```python
from build123d import *

# Parameters (mm, degrees)
SKETCH1_W           = 35
SKETCH1_H           = 48
BOSS_EXTRUDE1_DEPTH = 4
SKETCH2_W           = 35
SKETCH2_H           = 48
SKETCH2_W_2         = 31
SKETCH2_H_2         = 44
BOSS_EXTRUDE2_DEPTH = 5.5
SKETCH3_W           = 10
SKETCH3_H           = 6
SKETCH3_W_2         = 5.25
SKETCH3_H_2         = 8
BOSS_EXTRUDE3_DEPTH = 5.5
SKETCH4_W           = 20.5
SKETCH4_H           = 5.5
CUT_EXTRUDE1_DEPTH  = 3
CUT_EXTRUDE2_DEPTH  = 2
CUT_EXTRUDE3_REACH  = 33.185
SKETCH7_W           = 5.25
SKETCH7_H           = 3.1
CUT_EXTRUDE4_START  = 9.5
SKETCH8_R           = 1.55
CUT_EXTRUDE4_DEPTH  = 5.5
SKETCH5_W           = 5
SKETCH5_H           = 5
CUT_EXTRUDE5_DEPTH  = 2


with BuildPart() as part:
    # Sketch1 → Boss-Extrude1 (new body)
    with BuildSketch(Plane(origin=(0, 0, 0), x_dir=(1, 0, 0), z_dir=(0, 1, 0))):
        Rectangle(SKETCH1_W, SKETCH1_H)
    extrude(amount=BOSS_EXTRUDE1_DEPTH)

    # Sketch2 → Boss-Extrude2 (add)
    with BuildSketch(Plane(origin=(0, 4, 0), x_dir=(1, 0, 0), z_dir=(0, 1, 0))):
        Rectangle(SKETCH2_W, SKETCH2_H)
        with Locations((0, 1)):
            Rectangle(SKETCH2_W_2, SKETCH2_H_2, mode=Mode.SUBTRACT)
    extrude(amount=BOSS_EXTRUDE2_DEPTH)

    # Sketch3 → Boss-Extrude3 (add)
    with BuildSketch(Plane(origin=(0, 4, 0), x_dir=(1, 0, 0), z_dir=(0, 1, 0))):
        with Locations((0, 20)):
            Rectangle(SKETCH3_W, SKETCH3_H)
        with Locations((-12.875, -17)):
            Rectangle(SKETCH3_W_2, SKETCH3_H_2)
        with Locations((12.875, -17)):
            Rectangle(SKETCH3_W_2, SKETCH3_H_2)
    extrude(amount=BOSS_EXTRUDE3_DEPTH)

    # Sketch4 → Cut-Extrude1 (cut)
    with BuildSketch(Plane.XY.offset(24)):
        with Locations((0, 6.75)):
            Rectangle(SKETCH4_W, SKETCH4_H)
    extrude(amount=-CUT_EXTRUDE1_DEPTH, mode=Mode.SUBTRACT)

    # Sketch6 → Cut-Extrude2 (cut)
    with BuildSketch(Plane(origin=(0, 0, -24), x_dir=(-1, 0, 0), z_dir=(0, 0, -1))):
        with BuildLine():
            ThreePointArc((-12.93428015, 9.5), (-10, 5.4), (-7.06571985, 9.5))
            Line((-7.06571985, 9.5), (-12.93428015, 9.5))
        make_face()
        with BuildLine():
            Line((12.93428015, 9.5), (7.06571985, 9.5))
            ThreePointArc((7.06571985, 9.5), (10, 5.4), (12.93428015, 9.5))
        make_face()
    extrude(amount=-CUT_EXTRUDE2_DEPTH, mode=Mode.SUBTRACT)

    # Cut-Extrude3: up to this face of the body (flat: up to its plane)
    cut_extrude3_end = Plane(part.part.faces().sort_by_distance((0, 0, 0))[0])
    # Sketch7 → Cut-Extrude3 (cut, up to the picked face)
    with BuildSketch(Plane(origin=(0, 9.5, 0), x_dir=(1, 0, 0), z_dir=(0, 1, 0)), mode=Mode.PRIVATE) as cut_extrude3_sk1:
        with Locations((-12.875, -13.55)):
            Rectangle(SKETCH7_W, SKETCH7_H)
    cut_extrude3_tool1 = split(extrude(cut_extrude3_sk1.sketch, amount=-CUT_EXTRUDE3_REACH, mode=Mode.PRIVATE), bisect_by=cut_extrude3_end, keep=Keep.BOTH, mode=Mode.PRIVATE)
    add(cut_extrude3_tool1.solids().sort_by(Axis((-12.875, 9.5, 13.55), (0, -1, 0)))[0], mode=Mode.SUBTRACT)

    # Sketch8 → Cut-Extrude4 (cut)
    with BuildSketch(Plane(origin=(0, 0, 0), x_dir=(1, 0, 0), z_dir=(0, 1, 0)).offset(CUT_EXTRUDE4_START)):
        with Locations(Location((-12.55, -17.7, 0), (0, 0, 270))):
            Circle(SKETCH8_R)
        with Locations(Location((12.55, -17.7, 0), (0, 0, 270))):
            Circle(SKETCH8_R)
        with Locations(Location((0, 19.6, 0), (0, 0, 270))):
            Circle(SKETCH8_R)
    extrude(amount=-CUT_EXTRUDE4_DEPTH, mode=Mode.SUBTRACT)

    # Sketch5 → Cut-Extrude5 (cut)
    with BuildSketch(Plane.XZ):
        with Locations((-0.05, 6.1)):
            Rectangle(SKETCH5_W, SKETCH5_H)
        with Locations((-0.05, -6.1)):
            Rectangle(SKETCH5_W, SKETCH5_H)
    extrude(amount=-CUT_EXTRUDE5_DEPTH, mode=Mode.SUBTRACT)


solid = part.part
```
Design review of the part built by this model. Coordinates are the model's own, in mm. A direction names the side the tool comes from. Give positions to 0.01 mm unless a question says otherwise; leave off trailing zeros. Order: outer loops, then holes, each group sorted by start corner. A loop starts at its lowest first (then second) coordinate and runs counter-clockwise, first axis right, second up. Notation, with made-up numbers: (-13, 0.25) -> (-7, 0.25) arc R38 ccw to (-7, 38.25) -> close; hole circle Ø4 at (-6, 74). An arc over 180 degrees is marked (long way). Write each question's results on one line, items separated by ' | '. Start each with the question number.
Q1. Add section A-A on z = 14. Give the boundary of the cut face in (x, y).
Q2. Mouldability with a two-part tool opening along Z and no side actions: class faces 1 (the cylindrical face through (-9.9, 5.4, -23.5)), 2 (the cylindrical face through (-0.594, 6.788, -18.168)) as +Z half, -Z half, draft (parallel to the pull), parting line (faces both ways), or undercut.
Q3. Add section C-C on x = -15. Give the boundary of the cut face in (y, z).
Q4. Machinability: for faces 3 (the flat face through (10.25, 7, 19)), 4 (the flat face through (13, 7, 13)), 5 (the flat face through (0, 2, -6)), 6 (the cylindrical face through (10.1, 5.4, -23.5)), 7 (the flat face through (-13, 5, 15.1)), which of the approach directions +Z, -Z, +X, -X, +Y, -Y give a long, thin tool a straight path to every point of the face, cutting with its end or side? Answer none if there is none.
Q5. For pin 1 (2.5 mm diameter, centred on x = -12.5, z = 17.5, fed in from +Y); pin 2 (2 mm diameter, centred on x = -8.5, y = 8, fed in from -Z), all flat-tipped, find the tip position at first contact; note any pin that passes through.
Q6. Add section B-B on y = 7.75. Give the boundary of the cut face in (x, z).
Q7. Add section D-D on y = 1. Give the boundary of the cut face in (x, z), and give its area (3 significant figures).
Q8. Wall thickness on L1, parallel to X at y = 7.75, z = 17.7; L2, parallel to X at y = 8.5, z = -23.45; L3, parallel to Z at x = -12.5, y = 4.5: over which ranges is each line inside the solid? List them lowest first. Write a range as from..to.
Found:
1) outline: (-17.5, 0) -> (-15.5, 0) -> (-15.5, 9.5) -> (-17.5, 9.5) -> close; (-10.25, 0) -> (17.5, 0) -> (17.5, 9.5) -> (10.25, 9.5) -> (10.25, 4) -> (-10.25, 4) -> close
2) face 1: draft | face 2: undercut
3) outline: (0, -24) -> (9.5, -24) -> (9.5, -23) -> (4, -23) -> (4, 12) -> (0, 12) -> close; (0, 15.1) -> (9.5, 15.1) -> (9.5, 24) -> (0, 24) -> close
4) face 3: +Z, +Y | face 4: +Y | face 5: -Y | face 6: -Z | face 7: +Y, -Y
5) pin 1: stops at y = 4 | pin 2: passes through
6) outline: (-17.5, -24) -> (-13.01, -24) -> (-13.01, -23) -> (-15.5, -23) -> (-15.5, 15.1) -> (-10.25, 15.1) -> (-10.25, 24) -> (-17.5, 24) -> close; (-6.99, -24) -> (6.99, -24) -> (6.99, -23) -> (5, -23) -> (5, -17) -> (-5, -17) -> (-5, -23) -> (-6.99, -23) -> close; (10.25, 13) -> (15.5, 13) -> (15.5, -23) -> (13.01, -23) -> (13.01, -24) -> (17.5, -24) -> (17.5, 24) -> (10.25, 24) -> close; hole circle Ø3.1 at (-12.55, 17.7); hole circle Ø3.1 at (0, -19.6); hole circle Ø3.1 at (12.55, 17.7)
7) outline: (-17.5, -24) -> (17.5, -24) -> (17.5, 24) -> (-17.5, 24) -> close; hole (-15.5, 12) -> (-10.25, 12) -> (-10.25, 15.1) -> (-15.5, 15.1) -> close; hole (-2.55, -8.6) -> (2.45, -8.6) -> (2.45, -3.6) -> (-2.55, -3.6) -> close; hole (-2.55, 3.6) -> (2.45, 3.6) -> (2.45, 8.6) -> (-2.55, 8.6) -> close | area: 1,610 mm2
8) L1: x = -17.5..-14.1, -11..-10.25, 10.25..11, 14.1..17.5 | L2: x = -17.5..-13.1, -6.9..6.9, 13.1..17.5 | L3: z = -24..-23, 15.1..16.15, 19.25..24
